For this review, use the dimensioned drawing (mm, ordinates from the lowest corner) and the shaded views. A direction names the side the tool comes from. Give positions to 0.01 mm unless a question says otherwise; leave off trailing zeros. Loops run counter-clockwise (first coordinate to the right, second up) from the corner with the lowest first, then second, coordinate; pieces in that order, holes last. Notation, with made-up numbers: M 12.25,49.25 L 66.25,49.25 A7 ccw 66.25,57.25 Z; hole C 18.25,13.5 d3. An arc over 180 degrees is marked long. Use a Markdown table: item, result. Add a question column.
(1) Add section C-C, the plane z = 3.75. Give the boundary of the cut face in (x, y), then the cut area to 3 significant figures.
(2) Add section B-B, the plane z = 2.8. Give the boundary of the cut face in (x, y).
(3) Draft analysis for pull direction Y (two halves, no side actions). For the marked faces 3, 4 and 5, state which applies: pulls with the +Y half, pulls with the -Y half, needs draft (parallel to the pull), parting line crosses it, or undercut.
(4) For the marked faces 1 and 2, list the 3-axis set-ups (+Z, -Z, +X, -X, +Y, -Y) from which the entire face can be reached by the end or side of a thin tool; tool diameter is ignored.
(5) Add section A-A, the plane z = 0.4. Give the boundary of the cut face in (x, y), then the cut area to 3 significant figures.
(6) Insertion check: pin 1 Ø1.5 at (y, z) = (3.5, 2) entering from +X; pin 2 Ø1.5 at (y, z) = (12, 1.5) entering from +X; pin 3 Ø1 at (x, y) = (5, 6) entering from -Z. Each pin has a flat end and moves straight along its axis. Give the tip position at first contact, or say it passes through.
(7) For probe 1 along Y at (x, z) = (8, 0.4); probe 2 along Y at (x, z) = (4.5, 0.95); probe 3 along X at (y, z) = (11.75, 0.25), list the stretches that pass through material, from the lowest coordinate up.
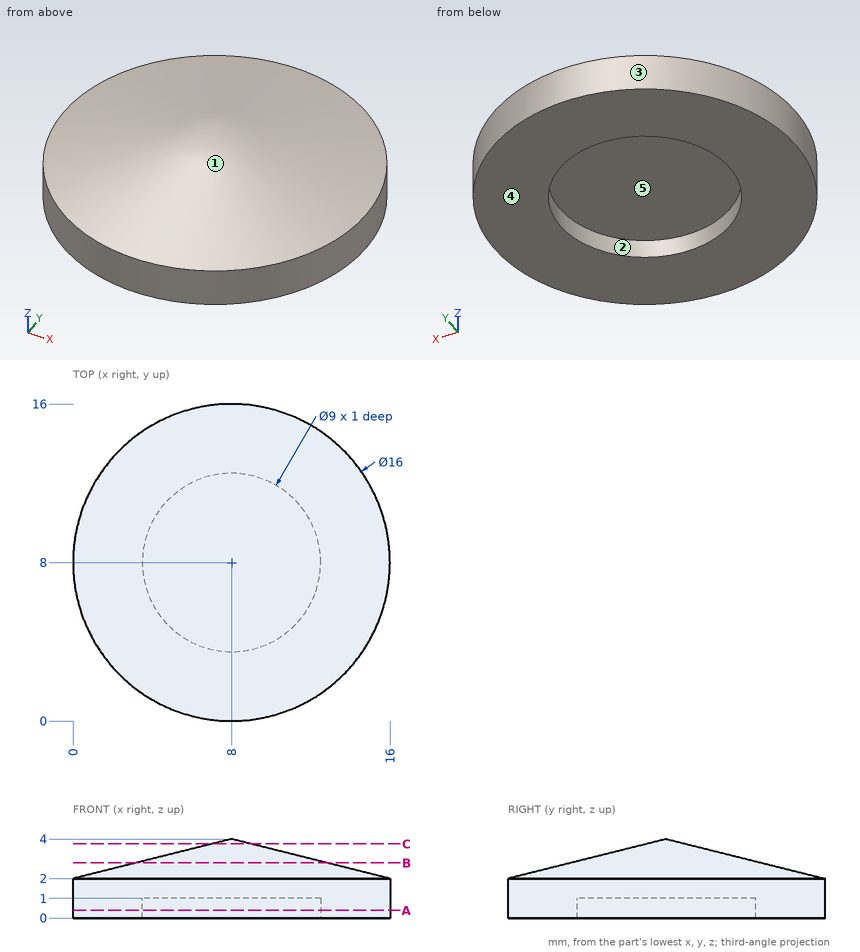
Established:
| question | item | result |
|---|---|---|
| 1 | outline | C 8,8 d2 |
| 1 | area | 3.14 mm^2 |
| 2 | outline | C 8,8 d9.6 |
| 3 | face 3 | parting line crosses it |
| 3 | face 4 | needs draft |
| 3 | face 5 | undercut |
| 4 | face 1 | +Z |
| 4 | face 2 | -Z |
| 5 | outline | C 8,8 d16; hole C 8,8 d9 |
| 5 | area | 137 mm^2 |
| 6 | pin 1 | x = 15.07 |
| 6 | pin 2 | x = 15.31 |
| 6 | pin 3 | z = 1 |
| 7 | probe 1 | 0 to 3.5, 12.5 to 16 |
| 7 | probe 2 | 0.81 to 5.17, 10.83 to 15.19 |
| 7 | probe 3 | 0.93 to 5.51, 10.49 to 15.07 |
